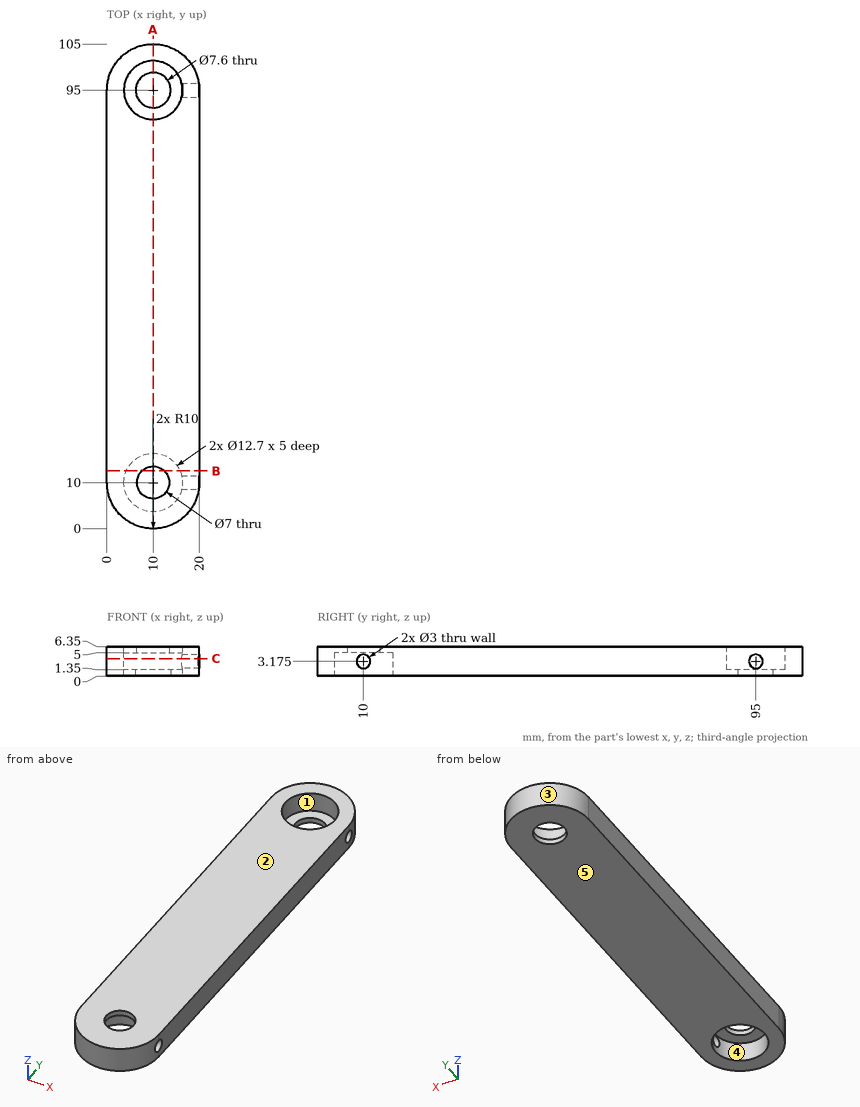
Design review of the part shown in the three views and the two pictorial views. Dimensions are in mm from the part's minimum x, y and z. A direction names the side the tool comes from. Give positions to 0.01 mm unless a question says otherwise; leave off trailing zeros. Loops run counter-clockwise (first coordinate to the right, second up) from the corner with the lowest first, then second, coordinate; pieces in that order, holes last. Notation, with made-up numbers: (56, -8) -> (114, -8) arc R23 cw to (114, 13) -> close; hole circle Ø11 at (3, -24.5). An arc over 180 degrees is marked (long way). Answer as a JSON object with one key per item and string values. Group by question number.
Q1. Tool access review of the marked faces 1 and 2: name each direction out of +Z, -Z, +X, -X, +Y, -Y from which nothing blocks a thin tool from reaching the whole face with its end or side.
Q2. Take a section at B-B (y = 12.5). Write out the cut boundary in (x, z), plus the area to 3 significant figures.
Q3. Insertion check: pin 1 (7.5 mm diameter, centred on x = 10, y = 95, fed in from +Z); pin 2 (1.8 mm diameter, centred on y = 95, z = 3.175, fed in from +X); pin 3 (4 mm diameter, centred on x = 12.5, y = 95.5, fed in from +Z); pin 4 (3 mm diameter, centred on x = 17.5, z = 1, fed in from +Y). Each pin has a flat end and moves straight along its axis. Give the tip position at first contact, or say it passes through.
Q4. Draft analysis for pull direction X (two halves, no side actions). For the marked faces 3, 4 and 5, state which applies: pulls with the +X half, pulls with the -X half, needs draft (parallel to the pull), parting line crosses it, or undercut.
Q5. Wall thickness on line 1 along Y through (x, z) = (10, 5.1); line 2 along Y through (x, z) = (6.75, 2.25); line 3 along Z through (x, y) = (12, 100.5): over which ranges is each line inside the solid? List them lowest first.
Q6. Take a section at A-A (x = 10). Write out the cut boundary in (y, z).
Q7. Take a section at C-C (z = 3.75). Write out the cut boundary in (x, y), plus the area to 3 significant figures.
Answer below:
{
 "1": {"face 1": "+Z", "face 2": "+Z, +X, -X, +Y, -Y"},
 "2": {"outline": "(0, 0) -> (4.16, 0) -> (4.16, 5) -> (7.55, 5) -> (7.55, 6.35) -> (0, 6.35) -> close; (12.45, 5) -> (15.84, 5) -> (15.84, 0) -> (20, 0) -> (20, 6.35) -> (12.45, 6.35) -> close", "area": "62.0 mm2"},
 "3": {"pin 1": "passes through", "pin 2": "stops at x = 3.71", "pin 3": "stops at z = 1.35", "pin 4": "stops at y = 103"},
 "4": {"face 3": "parting line crosses it", "face 4": "undercut", "face 5": "needs draft"},
 "5": {"line 1": "y = 0 to 6.5, 13.5 to 88.65, 101.35 to 105", "line 2": "y = 0.54 to 4.54, 15.46 to 89.54, 100.46 to 104.46", "line 3": "z = 0 to 1.35"},
 "6": {"outline": "(0, 0) -> (3.65, 0) -> (3.65, 5) -> (6.5, 5) -> (6.5, 6.35) -> (0, 6.35) -> close; (13.5, 5) -> (16.35, 5) -> (16.35, 0) -> (91.2, 0) -> (91.2, 1.35) -> (88.65, 1.35) -> (88.65, 6.35) -> (13.5, 6.35) -> close; (98.8, 0) -> (105, 0) -> (105, 6.35) -> (101.35, 6.35) -> (101.35, 1.35) -> (98.8, 1.35) -> close"},
 "7": {"outline": "(0, 10) arc R10 ccw to (19.9, 8.61) -> (16.2, 8.61) arc R6.35 cw (long way) to (16.2, 11.39) -> (20, 11.39) -> (20, 93.61) -> (16.2, 93.61) arc R6.35 cw (long way) to (16.2, 96.39) -> (19.9, 96.39) arc R10 ccw to (0, 95) -> close", "area": "1,740 mm2"}
}
